```python
from build123d import *

# Parameters (mm, degrees)
JOINT_BODY_DEPTH      = 5
JOINT_BODY_DEPTH_BACK = 5
ESQUISSE1_W           = 8
ESQUISSE1_H           = 6.5
ESQUISSE2_R           = 3.7
BEARINGHOLE_DEPTH     = 3.2
ESQUISSE4_W           = 8
ESQUISSE4_H           = 10
LOCKEREXTRUDE_DEPTH   = 3
ESQUISSE5_R           = 2.25
AXEHOLE_DEPTH         = 16
ESQUISSE6_W           = 7
ESQUISSE6_H           = 3
LOCKERHOLE_DEPTH      = 16
FIXATIONEXTRUDE_START = -5
FIXATIONEXTRUDE_DEPTH = 10
ESQUISSE8_R           = 1.6
FIXATIONHOLE_DEPTH    = 19.5
FIXATIONPROFILE_DEPTH = 27.419689627
CONG_1_R              = 3


with BuildPart() as part:
    # Esquisse1 → Joint body (new, two sides: drawn at the far end of the back side and taken through both)
    with BuildSketch(Plane.XY.offset(-JOINT_BODY_DEPTH_BACK)):
        with Locations((0, 10.463867403)):
            Rectangle(ESQUISSE1_W, ESQUISSE1_H)
    extrude(amount=JOINT_BODY_DEPTH + JOINT_BODY_DEPTH_BACK)

    # Esquisse2 → BearingHole (cut)
    with BuildSketch(Plane.XZ.offset(-7.213867403)):
        with Locations(Location((0, 0, 0), (0, 0, 270))):
            Circle(ESQUISSE2_R)
    extrude(amount=-BEARINGHOLE_DEPTH, mode=Mode.SUBTRACT)

    # Esquisse4 → LockerExtrude (add)
    with BuildSketch(Plane(origin=(0, 13.713867403, 0), x_dir=(1, 0, 0), z_dir=(0, 1, 0))):
        Rectangle(ESQUISSE4_W, ESQUISSE4_H)
    extrude(amount=LOCKEREXTRUDE_DEPTH)

    # Esquisse5 → AxeHole (cut)
    with BuildSketch(Plane(origin=(0, 16.713867403, 0), x_dir=(1, 0, 0), z_dir=(0, 1, 0))):
        with Locations(Location((0, 0, 0), (0, 0, 270))):
            Circle(ESQUISSE5_R)
    extrude(amount=-AXEHOLE_DEPTH, mode=Mode.SUBTRACT)

    # Esquisse6 → LockerHole (cut)
    with BuildSketch(Plane.XY.offset(5)):
        with Locations((0, 13.563867403)):
            Rectangle(ESQUISSE6_W, ESQUISSE6_H)
    extrude(amount=-LOCKERHOLE_DEPTH, mode=Mode.SUBTRACT)

    # Esquisse7 → FixationExtrude (add)
    with BuildSketch(Plane.XY.offset(FIXATIONEXTRUDE_START)):
        Polygon((12, -6.286132597), (10.743640135, 7.188023114), (4, 16.713867403), (4, 7.213867403), (5.258769643, -6.286132597), align=None)
    fixationextrude = extrude(amount=FIXATIONEXTRUDE_DEPTH)

    # Esquisse8 → FixationHole (cut)
    with BuildSketch(Plane.XZ.offset(6.286132597)):
        with Locations((9, 0)):
            Circle(ESQUISSE8_R)
    fixationhole = extrude(amount=-FIXATIONHOLE_DEPTH, mode=Mode.SUBTRACT)

    # Esquisse10 → FixationProfile (cut, through all)
    with BuildSketch(Plane.XZ.offset(6.286132597)):
        Polygon((12, 2.3), (12, 5), (4, 5), align=None)
        Polygon((12, -2.3), (12, -5), (4, -5), align=None)
    fixationprofile = extrude(amount=-FIXATIONPROFILE_DEPTH, mode=Mode.SUBTRACT)

    # Symétrie3: FixationExtrude, FixationHole, FixationProfile across plane
    add(fixationextrude.mirror(Plane(origin=(0, 0, 0), x_dir=(0, 0, 1), z_dir=(1, 0, 0))))
    add(fixationhole.mirror(Plane(origin=(0, 0, 0), x_dir=(0, 0, 1), z_dir=(1, 0, 0))), mode=Mode.SUBTRACT)
    add(fixationprofile.mirror(Plane(origin=(0, 0, 0), x_dir=(0, 0, 1), z_dir=(1, 0, 0))), mode=Mode.SUBTRACT)

    # Congé1
    cong_1_edges = [part.edges().sort_by_distance(p)[0] for p in [
        (-4.629384821, 0.463867403, -4.787582623),
        (-4.629384821, 0.463867403, 4.787582623),
        (4.629384821, 0.463867403, 4.787582623),
        (4.629384821, 0.463867403, -4.787582623),
    ]]
    fillet(cong_1_edges, radius=CONG_1_R)


solid = part.part
```
For this review, take the finished solid that the model builds, in its own axes (mm). A direction names the side the tool comes from. Coordinates: 2 decimals unless noted, no trailing zeros. Write each loop counter-clockwise with the first axis right and the second up, starting at its lowest first coordinate (ties: lowest second). Pieces come first, ordered by that corner, then holes.
(1) For pin 1 Ø1.5 at (y, z) = (14, 2.5) entering from +X; pin 2 Ø3.5 at (x, z) = (1, -2) entering from -Y; pin 3 Ø5 at (x, z) = (-3, 1) entering from -Y; pin 4 Ø1 at (x, z) = (0, 0.5) entering from +Y, all flat-tipped, find the tip position at first contact; note any pin that passes through.
(2) Add section A-A on x = 0. Give the boundary of the cut face in (y, z), then the cut area to 3 significant figures.
(3) Add section B-B on z = 0. Count the separate pieces of the cut face and the enclosed holes in it, then the cut area to 3 significant figures.
(4) Wall thickness on probe 1 along X at (y, z) = (-0.5, 0); probe 2 along Y at (x, z) = (-1.25, -3.75); probe 3 along X at (y, z) = (1, 1.25): over which ranges is each line inside the solid? List them lowest first.
(5) Add section D-D on x = 9.75. Give the boundary of the cut face in (y, z), then the cut area to 3 significant figures.
(6) Add section C-C on y = 9. Give the boundary of the cut face in (x, z), then the cut area to 3 significant figures.
(7) Tool access review of faces 4 (the face through (7.4, 0.7, 0.07)), 5 (the face through (0, 11, 5)), 6 (the face through (-2, 10.414, -2)), 7 (the face through (-0.8, 15.064, 2.3)), 8 (the face through (4.48, 2.06, -0.01)): name each direction out of +Z, -Z, +X, -X, +Y, -Y from which nothing blocks a thin tool from reaching the whole face with its end or side.
(8) The part is to be moulded in two halves that separate along Y. For faces 1 (the face through (-3.5, 14, 0)), 2 (the face through (-0.9, 16.714, -2.3)), 3 (the face through (-4.48, 2.06, -0.01)), say which applies: +Y half, -Y half, draft (parallel to the pull), parting line (faces both ways), or undercut.
Answer sheet:
1. pin 1: stops at x = 6.45
1. pin 2: stops at y = 7.21
1. pin 3: stops at y = -6.29
1. pin 4: passes through
2. outline: (7.21, -5) - (12.06, -5) - (12.06, -2.25) - (10.41, -2.25) - (10.41, -3.7) - (7.21, -3.7) - close; (7.21, 3.7) - (10.41, 3.7) - (10.41, 2.25) - (12.06, 2.25) - (12.06, 5) - (7.21, 5) - close; (15.06, -5) - (16.71, -5) - (16.71, -2.25) - (15.06, -2.25) - close; (15.06, 2.25) - (16.71, 2.25) - (16.71, 5) - (15.06, 5) - close
2. area: 26.5 mm2
3. separate pieces: 4
3. enclosed holes: 0
3. area: 160 mm2
4. probe 1: x = -11.46 to -10.6, -7.4 to -4.72, 4.72 to 7.4, 10.6 to 11.46
4. probe 2: y = 7.21 to 12.06, 15.06 to 16.71
4. probe 3: x = -11.32 to -10, -8 to -4.64, 4.64 to 8, 10 to 11.32
5. outline: (-6.29, -3.06) - (8.59, -3.06) - (8.59, -1.41) - (-6.29, -1.41) - close; (-6.29, 1.41) - (8.59, 1.41) - (8.59, 3.06) - (-6.29, 3.06) - close
5. area: 49.0 mm2
6. outline: (-9.46, -3.16) - (-4, -5) - (4, -5) - (9.46, -3.16) - (9.46, -1.53) arc R1.6 cw (long way) to (9.46, 1.53) - (9.46, 3.16) - (4, 5) - (-4, 5) - (-9.46, 3.16) - (-9.46, 1.53) arc R1.6 cw (long way) to (-9.46, -1.53) - close; hole circle Ø7.4 at (0, 0)
6. area: 115 mm2
7. face 4: +Y, -Y
7. face 5: +Z, +X, -X, +Y, -Y
7. face 6: -Y
7. face 7: +Z, -Z
7. face 8: +Z, -Z, -Y
8. face 1: undercut
8. face 2: +Y half
8. face 3: -Y half
